Geometry check sheet. Reference: the model listing, model coordinates, mm. Face numbers are marked on the shaded views. A direction names the side the tool comes from. Coordinates: 2 decimals unless noted, no trailing zeros. Write each loop counter-clockwise with the first axis right and the second up, starting at its lowest first coordinate (ties: lowest second). Pieces come first, ordered by that corner, then holes.
from build123d import *

# Parameters (mm, degrees)
SKETCH1_R           = 27.7
BOSS_EXTRUDE1_DEPTH = 3
SKETCH2_R           = 11
CUT_EXTRUDE1_DEPTH  = 2
SKETCH4_R           = 10
CUT_EXTRUDE2_DEPTH  = 3
SKETCH5_R           = 12.1
BOSS_EXTRUDE3_DEPTH = 3
SKETCH6_W           = 10
SKETCH6_H           = 27.7
CUT_EXTRUDE3_DEPTH  = 3
BOSS_EXTRUDE4_DEPTH = 5


with BuildPart() as part:
    # Sketch1 → Boss-Extrude1 (new body)
    with BuildSketch(Plane.XY):
        Circle(SKETCH1_R)
    extrude(amount=BOSS_EXTRUDE1_DEPTH)

    # Sketch2 → Cut-Extrude1 (cut)
    with BuildSketch(Plane.XY.offset(3)):
        with Locations((-10.394469683, -10.394469683)):
            Circle(SKETCH2_R)
        with Locations((10.394469683, 10.394469683)):
            Circle(SKETCH2_R)
    extrude(amount=-CUT_EXTRUDE1_DEPTH, mode=Mode.SUBTRACT)

    # Sketch4 → Cut-Extrude2 (cut)
    with BuildSketch(Plane.XY.offset(3)):
        Circle(SKETCH4_R)
    extrude(amount=-CUT_EXTRUDE2_DEPTH, mode=Mode.SUBTRACT)

    # Sketch6 → Cut-Extrude3 (cut)
    with BuildSketch(Plane.XY.offset(3)):
        with Locations((0, -13.85)):
            Rectangle(SKETCH6_W, SKETCH6_H)
    extrude(amount=-CUT_EXTRUDE3_DEPTH, mode=Mode.SUBTRACT)



with BuildPart() as body_2:
    # Sketch5 → Boss-Extrude3 (new body)
    with BuildSketch(Plane.XY.offset(3)):
        with BuildLine():
            Line((-27.7, 0), (-27.7, 62.5))
            Line((-27.7, 62.5), (27.7, 62.5))
            Line((27.7, 62.5), (27.7, 0))
            ThreePointArc((27.7, 0), (0, 27.7), (-27.7, 0))
        make_face()
        with Locations((0, 49)):
            Circle(SKETCH5_R, mode=Mode.SUBTRACT)
    extrude(amount=-BOSS_EXTRUDE3_DEPTH)


with BuildPart() as part_1:
    add(part.part)

    add(body_2.part)  # Boss-Extrude4 merges body 2
    # Sketch8 → Boss-Extrude4 (add)
    with BuildSketch(Plane(origin=(0, 0, 0), x_dir=(-1, 0, 0), z_dir=(0, 0, -1))):
        with BuildLine():
            Line((-23.7, 62.5), (23.7, 62.5))
            Line((23.7, 62.5), (25.7, 62.5))
            Line((25.7, 62.5), (25.7, 0))
            ThreePointArc((25.7, 0), (19.863362581, -16.32329625), (5, -25.244999541))
            Line((5, -25.244999541), (5, -23.244999541))
            ThreePointArc((5, -23.244999541), (18.444726934, -14.91660152), (23.7, 0))
            Line((23.7, 0), (23.7, 61.1))
            Line((23.7, 61.1), (-23.7, 61.1))
            Line((-23.7, 61.1), (-23.7, 0))
            ThreePointArc((-23.7, 0), (-18.444726934, -14.91660152), (-5, -23.244999541))
            Line((-5, -23.244999541), (-5, -25.244999541))
            ThreePointArc((-5, -25.244999541), (-19.863362581, -16.32329625), (-25.7, 0))
            Line((-25.7, 0), (-25.7, 62.5))
            Line((-25.7, 62.5), (-23.7, 62.5))
        make_face()
    extrude(amount=BOSS_EXTRUDE4_DEPTH)


solid = part_1.part
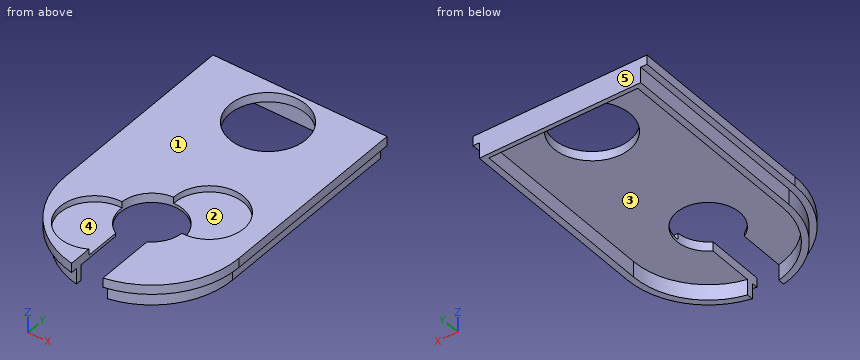
1. Gauge pin test, flat ends, axial feed: pin 1 Ø8 at (x, y) = (12, 16.5) entering from +Z; pin 2 Ø6 at (x, y) = (4, -10) entering from -Z; pin 3 Ø25 at (x, y) = (12, 3.5) entering from -Z; pin 4 Ø2.5 at (y, z) = (23, -3.5) entering from +X. Record the tip position at first contact, or that the pin passes through.
Computed values:
pin 1: stops at z = 1
pin 2: stops at z = 0
pin 3: stops at z = -5
pin 4: stops at x = 25.7
2. Thickness scan on line 1 along X through (y, z) = (50, -1.5); line 2 along Z through (x, y) = (-1.5, 26); line 3 along X through (y, z) = (-17, 1.75). Record the ranges inside material, lowest first.
Computed values:
line 1: x = -25.7 to -23.7, 23.7 to 25.7
line 2: z = 0 to 3
line 3: x = -21.87 to -19.19, 5 to 21.87
3. Sectioned sample at A-A, the plane y = 49. Record the boundary of the cut face in (x, z), and give its area (3 significant figures).
Computed values:
outline: (-27.7, 0) - (-25.7, 0) - (-25.7, -5) - (-23.7, -5) - (-23.7, 0) - (-12.1, 0) - (-12.1, 3) - (-27.7, 3) - close; (12.1, 0) - (23.7, 0) - (23.7, -5) - (25.7, -5) - (25.7, 0) - (27.7, 0) - (27.7, 3) - (12.1, 3) - close
area: 114 mm2
4. Sectioned sample at B-B, the plane y = 34. Record the boundary of the cut face in (x, z).
Computed values:
outline: (-27.7, 0) - (-25.7, 0) - (-25.7, -5) - (-23.7, -5) - (-23.7, 0) - (23.7, 0) - (23.7, -5) - (25.7, -5) - (25.7, 0) - (27.7, 0) - (27.7, 3) - (-27.7, 3) - close
5. Sectioned sample at C-C, the plane z = -2. Record the boundary of the cut face in (x, y) (3 decimals).
Computed values:
outline: (-25.7, 0) arc R25.744 ccw to (-5, -25.245) - (-5, -23.245) arc R23.797 cw to (-23.7, 0) - (-23.7, 61.1) - (23.7, 61.1) - (23.7, 0) arc R23.797 cw to (5, -23.245) - (5, -25.245) arc R25.744 ccw to (25.7, 0) - (25.7, 62.5) - (-25.7, 62.5) - close
6. Sectioned sample at D-D, the plane x = -3.5. Record the boundary of the cut face in (y, z), and give its area (3 significant figures).
Computed values:
outline: (9.37, 0) - (37.42, 0) - (37.42, 3) - (9.37, 3) - close; (60.58, 0) - (61.1, 0) - (61.1, -5) - (62.5, -5) - (62.5, 3) - (60.58, 3) - close
area: 96.9 mm2
7. Draft check along X on the marked faces 3, 4 and 5. Enter one of: released by +X, released by -X, zero draft, split by the parting line, or undercut.
Computed values:
face 3: undercut
face 4: undercut
face 5: zero draft
8. Access from +Z, -Z, +X, -X, +Y, -Y to the whole of each face (thin tool, end or side, straight path). Record for the marked faces 1 and 2.
Computed values:
face 1: +Z, +X, -X, +Y, -Y
face 2: +Z
